from build123d import *

# Parameters (mm, degrees)
SKETCH_1_W          = 477
SKETCH_1_H          = 188
EXTRUDE_1_DEPTH     = 3
SKETCH_2_R          = 1.5
SKETCH_2_R_2        = 1.502344372
CUT_EXTRUDE_1_DEPTH = 257.373263037
CUT_EXTRUDE_3_DEPTH = 10
SKETCH_3_W          = 39
SKETCH_3_H          = 144
CUT_EXTRUDE_4_DEPTH = 10
FILLET_1_R          = 10
FILLET_2_R          = 3


with BuildPart() as part:
    # 草图1 → 凸台-拉伸1 (new body)
    with BuildSketch(Plane.XY):
        Rectangle(SKETCH_1_W, SKETCH_1_H)
    extrude(amount=EXTRUDE_1_DEPTH)

    # 草图2 → 切除-拉伸1 (cut, through all)
    with BuildSketch(Plane.XY.offset(3)):
        with Locations((228.5, 84)):
            Circle(SKETCH_2_R)
        with Locations((-228.5, 84)):
            Circle(SKETCH_2_R)
        with Locations((-228.5, -84)):
            Circle(SKETCH_2_R)
        with Locations((228.5, -84)):
            Circle(SKETCH_2_R)
        with Locations((207.5, -84)):
            Circle(SKETCH_2_R_2)
        with Locations(Location((207.5, 84, 0), (0, 0, 180))):
            Circle(SKETCH_2_R_2)
        with Locations(Location((-207.5, -84, 0), (0, 0, 180))):
            Circle(SKETCH_2_R_2)
        with Locations((-207.5, 84)):
            Circle(SKETCH_2_R_2)
    extrude(amount=-CUT_EXTRUDE_1_DEPTH, mode=Mode.SUBTRACT)

    # 草图4 → 切除-拉伸3 (cut)
    with BuildSketch(Plane.XY.offset(3)):
        with BuildLine():
            Line((-231, 85.5), (-226, 85.5))
            ThreePointArc((-226, 85.5), (-224.5, 84), (-226, 82.5))
            Line((-226, 82.5), (-231, 82.5))
            ThreePointArc((-231, 82.5), (-232.5, 84), (-231, 85.5))
        make_face()
        with BuildLine():
            Line((-210, 85.5), (-205, 85.5))
            ThreePointArc((-205, 85.5), (-203.5, 84), (-205, 82.5))
            Line((-205, 82.5), (-210, 82.5))
            ThreePointArc((-210, 82.5), (-211.5, 84), (-210, 85.5))
        make_face()
        with BuildLine():
            Line((231, 85.5), (226, 85.5))
            ThreePointArc((226, 85.5), (224.5, 84), (226, 82.5))
            Line((226, 82.5), (231, 82.5))
            ThreePointArc((231, 82.5), (232.5, 84), (231, 85.5))
        make_face()
        with BuildLine():
            Line((210, 85.5), (205, 85.5))
            ThreePointArc((205, 85.5), (203.5, 84), (205, 82.5))
            Line((205, 82.5), (210, 82.5))
            ThreePointArc((210, 82.5), (211.5, 84), (210, 85.5))
        make_face()
    cut_extrude_3 = extrude(amount=-CUT_EXTRUDE_3_DEPTH, mode=Mode.SUBTRACT)

    # 镜向1: 切除-拉伸3 across plane
    add(cut_extrude_3.mirror(Plane.ZX), mode=Mode.SUBTRACT)

    # 草图3 → 切除-拉伸4 (cut)
    with BuildSketch(Plane.XY.offset(3)):
        with Locations((219, 0)):
            Rectangle(SKETCH_3_W, SKETCH_3_H)
        with Locations((-219, 0)):
            Rectangle(SKETCH_3_W, SKETCH_3_H)
    extrude(amount=-CUT_EXTRUDE_4_DEPTH, mode=Mode.SUBTRACT)

    # 圆角1
    fillet_1_edges = [part.edges().sort_by_distance(p)[0] for p in [
        (199.5, -72, 1.5),
        (199.5, 72, 1.5),
        (-199.5, 72, 1.5),
        (-199.5, -72, 1.5),
    ]]
    fillet(fillet_1_edges, radius=FILLET_1_R)

    # 圆角2
    fillet_2_edges = [part.edges().sort_by_distance(p)[0] for p in [
        (-238.5, 72, 1.5),
        (-238.5, -72, 1.5),
        (238.5, 72, 1.5),
        (238.5, -72, 1.5),
        (238.5, -94, 1.5),
        (-238.5, -94, 1.5),
        (-238.5, 94, 1.5),
        (238.5, 94, 1.5),
    ]]
    fillet(fillet_2_edges, radius=FILLET_2_R)


solid = part.part
Input: part model. Units: mm. Frame: model coordinates. A direction names the side the tool comes from. Coordinates: 2 decimals unless noted, no trailing zeros. Loops run counter-clockwise (first coordinate to the right, second up) from the corner with the lowest first, then second, coordinate; pieces in that order, holes last.
Q1. Contact query for flat-ended pins moving along their axis: pin 1 (12 mm diameter, centred on x = -190.5, y = 73.5, fed in from -Z); pin 2 (1 mm diameter, centred on y = -24, z = 2, fed in from -X); pin 3 (0.9 mm diameter, centred on y = -22, z = 2, fed in from +X). Output: stop coordinate, or through.
Q2. Cut plane A-A (z = 1.35). Give the number of separate pieces and of enclosed holes in the cut face, then the cut area to 3 significant figures.
Q3. Set-up query: faces 3 (the face through (-3, 1, 3)), 4 (the face through (-202.35, 68.99, 1.48)), 5 (the face through (202.35, -68.99, 1.48)). Return all of +Z, -Z, +X, -X, +Y, -Y with unobstructed straight access to the full face (end or side cutting, diameter ignored); none if empty.
Q4. Draft query along Y for faces 1 (the face through (-202.51, -69.15, 1.48)), 2 (the face through (-3, 1, 0)). Return one class per face: +Y half, -Y half, draft (parallel to the pull), parting line (faces both ways), or undercut.
Q5. Material intervals for line 1 (X direction, y = -83.5, z = 0.5); line 2 (Y direction, x = -214, z = 1); line 3 (X direction, y = 19, z = 0.4), sorted ascending.
Q6. Cut plane B-B (y = -46). Output: boundary loops of the cut face in (x, z).
Working result:
1. pin 1: stops at z = 0
1. pin 2: stops at x = -199.5
1. pin 3: stops at x = 199.5
2. separate pieces: 1
2. enclosed holes: 8
2. area: 78,300 mm2
3. face 3: +Z, +X, -X, +Y, -Y
3. face 4: +Z, -Z, -X
3. face 5: +Z, -Z, +X
4. face 1: undercut
4. face 2: draft
5. line 1: x = -238.5 to -232.41, -224.59 to -211.41, -203.59 to 203.59, 211.41 to 224.59, 232.41 to 238.5
5. line 2: y = -94 to -72, 72 to 94
5. line 3: x = -199.5 to 199.5
6. outline: (-199.5, 0) - (199.5, 0) - (199.5, 3) - (-199.5, 3) - close
